Can you work these out from the model? Positions are in its coordinate system, mm. Face numbers are marked on the shaded views. Give positions to 0.01 mm unless a question says otherwise; leave off trailing zeros. Write each loop counter-clockwise with the first axis right and the second up, starting at its lowest first coordinate (ties: lowest second). Pieces come first, ordered by that corner, then holes. Notation, with made-up numbers: M -22,9.5 L 20,9.5 A23 ccw 20,34.5 Z; hole C 77.5,15.5 d6. An arc over 180 degrees is marked long. Write each question's results on one line, items separated by ' | '.
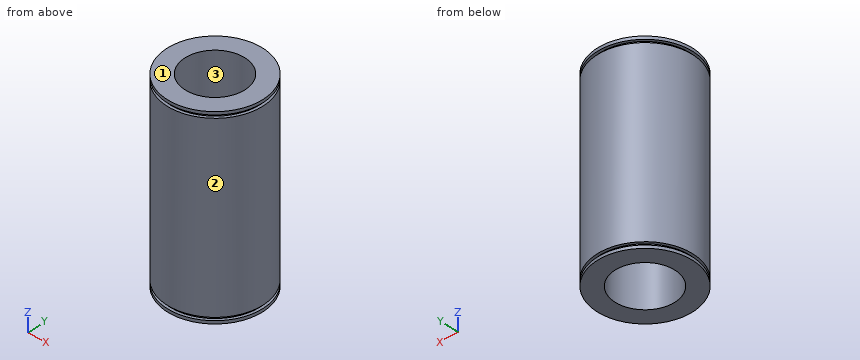
from build123d import *

# Parameters (mm, degrees)
SKETCH1_R           = 25.4
SKETCH1_R_2         = 15.875
BOSS_EXTRUDE1_DEPTH = 50.8
SKETCH2_W           = 1.5875
SKETCH2_H           = 1.4478


with BuildPart() as part:
    # Sketch1 → Boss-Extrude1 (new, symmetric)
    with BuildSketch(Plane.XY):
        Circle(SKETCH1_R)
        Circle(SKETCH1_R_2, mode=Mode.SUBTRACT)
    extrude(amount=BOSS_EXTRUDE1_DEPTH, both=True)

    # Sketch2 → Cut-Revolve1 (revolve, cut)
    with BuildSketch(Plane(origin=(0, 0, 0), x_dir=(0, 0, -1), z_dir=(1, 0, 0)), mode=Mode.PRIVATE) as cut_revolve1_sk:
        with Locations((-48.41875, 24.6761)):
            Rectangle(SKETCH2_W, SKETCH2_H)
    cut_revolve1 = revolve(cut_revolve1_sk.sketch.rotate(Axis((0, 0, 0), (0, 0, 1)), 90), axis=Axis((0, 0, 0), (0, 0, 1)), mode=Mode.SUBTRACT)

    # Mirror1: Cut-Revolve1 across plane
    add(cut_revolve1.mirror(Plane.XY), mode=Mode.SUBTRACT)


solid = part.part
Item 1: I'm going to push flat-ended pins straight in: pin 1 (6 mm diameter, centred on y = 9.5, z = -26.5, fed in from -X); pin 2 (12 mm diameter, centred on x = -2.5, z = -11.5, fed in from -Y); pin 3 (1.5 mm diameter, centred on y = 18.5, z = 28.5, fed in from +X). Where does each tip first touch, or does it pass through?
Geometry says:
pin 1: stops at x = -24.55 | pin 2: stops at y = -25.4 | pin 3: stops at x = 18.17
Item 2: If I drill on line 1 (Z direction, x = -12.5, y = 21) (1 decimal); line 2 (Y direction, x = -0.5, z = -29.5); line 3 (Y direction, x = 5, z = -3.5), over which ranges is the centre line in solid material (lowest first)? Write a range as from..to.
Geometry says:
line 1: z = -50.8..-49.2, -47.6..47.6, 49.2..50.8 | line 2: y = -25.4..-15.87, 15.87..25.4 | line 3: y = -24.9..-15.07, 15.07..24.9
Item 3: I want a section at A-A, the plane y = 0. Please give me the cut outline in (x, z) (1 decimal), and give its area (3 significant figures).
Geometry says:
outline: M -25.4,-50.8 L -15.9,-50.8 L -15.9,50.8 L -25.4,50.8 L -25.4,49.2 L -24,49.2 L -24,47.6 L -25.4,47.6 L -25.4,-47.6 L -24,-47.6 L -24,-49.2 L -25.4,-49.2 Z; M 15.9,-50.8 L 25.4,-50.8 L 25.4,-49.2 L 24,-49.2 L 24,-47.6 L 25.4,-47.6 L 25.4,47.6 L 24,47.6 L 24,49.2 L 25.4,49.2 L 25.4,50.8 L 15.9,50.8 Z | area: 1,930 mm2
Item 4: I want a section at C-C, the plane y = -20. Please give me the cut outline in (x, z) (1 decimal).
Geometry says:
outline: M -15.7,-50.8 L 15.7,-50.8 L 15.7,-49.2 L 13.2,-49.2 L 13.2,-47.6 L 15.7,-47.6 L 15.7,47.6 L 13.2,47.6 L 13.2,49.2 L 15.7,49.2 L 15.7,50.8 L -15.7,50.8 L -15.7,49.2 L -13.2,49.2 L -13.2,47.6 L -15.7,47.6 L -15.7,-47.6 L -13.2,-47.6 L -13.2,-49.2 L -15.7,-49.2 Z
Item 5: I want a section at D-D, the plane z = -18. Please give me the cut outline in (x, y) (3 decimals), and give its area (3 significant figures).
Geometry says:
outline: C 0,0 d50.8; hole C 0,0 d31.75 | area: 1,240 mm2
Item 6: Thinking about a two-plate mould opening in X: for the marked faces 1, 2 and 3, which applies, +X half, -X half, draft (parallel to the pull), parting line (faces both ways), or undercut?
Geometry says:
face 1: draft | face 2: parting line | face 3: undercut
